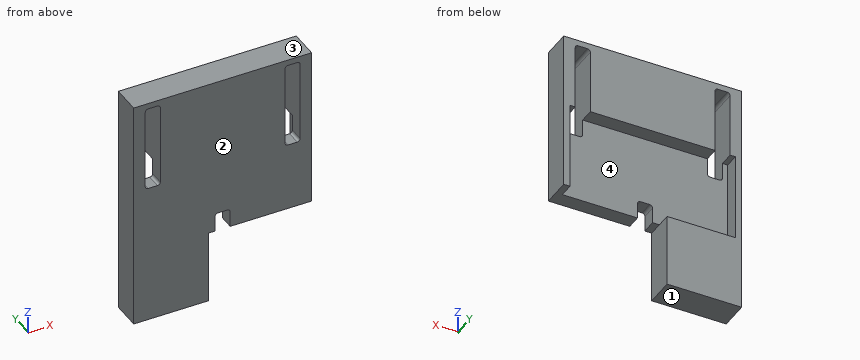
```python
from build123d import *

# Parameters (mm, degrees)
BOSS_EXTRUDE5_DEPTH = 10
CUT_EXTRUDE6_DEPTH  = 5
FILLET4_R           = 1
MIRROR25_DEPTH      = 10
MIRROR25_2_DEPTH    = 5
SKETCH20_W          = 35.925
SKETCH20_H          = 25.502594227
CUT_EXTRUDE7_DEPTH  = 10


# Read off the part's stored shape, not the designer's step: Mirror25
with BuildPart() as part:
    # Sketch15 → Boss-Extrude5 (new body)
    with BuildSketch(Plane(origin=(0, 0, 0), x_dir=(1, 0, 0), z_dir=(0, 1, 0))):
        Polygon((24.3, 76.900659127), (-6.625, 76.900659127), (-6.625, -4.5), (24.3, -4.5), (24.3, 44.900659127), (21.675, 44.900659127), (21.675, 47.400659127), (21.675, 72.400659127), (21.675, 74.900659127), (24.3, 74.900659127), align=None)
        Polygon((-2.625, 25), (-2.625, 0), (-2.625, -2.5), (0, -2.5), (2.625, -2.5), (2.625, 0), (2.625, 25), (2.625, 27.5), (0, 27.5), (-2.625, 27.5), align=None, mode=Mode.SUBTRACT)
    extrude(amount=BOSS_EXTRUDE5_DEPTH)

    # Sketch18 → Cut-Extrude6 (cut)
    with BuildSketch(Plane(origin=(0, 10, 0), x_dir=(1, 0, 0), z_dir=(0, 1, 0))):
        Polygon((21.675, 51.3980649), (-4.44053483, 51.3980649), (-4.44053483, 20.8980649), (24.3, 20.8980649), (24.3, 51.3980649), align=None)
    extrude(amount=-CUT_EXTRUDE6_DEPTH, mode=Mode.SUBTRACT)

    # Fillet4
    fillet4_edges = [part.edges().sort_by_distance(p)[0] for p in [
        (21.675, 5, -74.900659127),
        (-2.625, 5, 2.5),
        (2.625, 5, 2.5),
        (2.625, 2.5, -27.5),
        (-2.625, 2.5, -27.5),
        (21.675, 2.5, -44.900659127),
    ]]
    fillet(fillet4_edges, radius=FILLET4_R)

    # Mirror25 outline → Mirror25 (add)
    with BuildSketch(Plane(origin=(0, 0, 0), x_dir=(1, 0, 0), z_dir=(0, 1, 0))):
        with BuildLine():
            Line((45.975, 20.8980649), (24.3, 20.8980649))
            Line((24.3, 20.8980649), (24.3, -4.5))
            Line((24.3, -4.5), (55.225, -4.5))
            Line((55.225, -4.5), (55.225, 76.900659127))
            Line((55.225, 76.900659127), (24.3, 76.900659127))
            Line((24.3, 76.900659127), (24.3, 74.900659127))
            Line((24.3, 74.900659127), (25.925, 74.900659127))
            ThreePointArc((25.925, 74.900659127), (26.632106781, 74.607765908), (26.925, 73.900659127))
            Line((26.925, 73.900659127), (26.925, 51.3980649))
            Line((26.925, 51.3980649), (53.04053483, 51.3980649))
            Line((53.04053483, 51.3980649), (53.04053483, 20.8980649))
            Line((53.04053483, 20.8980649), (51.225, 20.8980649))
            Line((51.225, 20.8980649), (51.225, -1.5))
            ThreePointArc((51.225, -1.5), (50.932106781, -2.207106781), (50.225, -2.5))
            Line((50.225, -2.5), (46.975, -2.5))
            ThreePointArc((46.975, -2.5), (46.267893219, -2.207106781), (45.975, -1.5))
            Line((45.975, -1.5), (45.975, 20.8980649))
        make_face()
    extrude(amount=MIRROR25_DEPTH)

    # Mirror25 2 outline → Mirror25 2 (add)
    with BuildSketch(Plane(origin=(0, 0, 0), x_dir=(1, 0, 0), z_dir=(0, 1, 0))):
        with BuildLine():
            Line((25.925, 44.900659127), (24.3, 44.900659127))
            Line((24.3, 44.900659127), (24.3, 20.8980649))
            Line((24.3, 20.8980649), (45.975, 20.8980649))
            Line((45.975, 20.8980649), (45.975, 26.5))
            ThreePointArc((45.975, 26.5), (46.267893219, 27.207106781), (46.975, 27.5))
            Line((46.975, 27.5), (50.225, 27.5))
            ThreePointArc((50.225, 27.5), (50.932106781, 27.207106781), (51.225, 26.5))
            Line((51.225, 26.5), (51.225, 20.8980649))
            Line((51.225, 20.8980649), (53.04053483, 20.8980649))
            Line((53.04053483, 20.8980649), (53.04053483, 51.3980649))
            Line((53.04053483, 51.3980649), (26.925, 51.3980649))
            Line((26.925, 51.3980649), (26.925, 45.900659127))
            ThreePointArc((26.925, 45.900659127), (26.632106781, 45.193552346), (25.925, 44.900659127))
        make_face()
    extrude(amount=MIRROR25_2_DEPTH)

    # Sketch20 → Cut-Extrude7 (cut)
    with BuildSketch(Plane(origin=(0, 10, 0), x_dir=(1, 0, 0), z_dir=(0, 1, 0))):
        with Locations((37.2625, 64.149362014)):
            Rectangle(SKETCH20_W, SKETCH20_H)
    extrude(amount=-CUT_EXTRUDE7_DEPTH, mode=Mode.SUBTRACT)


solid = part.part
```
Could you check a few things on this model? Use its own coordinates, in mm. Face numbers are marked on the shaded views. Coordinates: 2 decimals unless noted, no trailing zeros. Write each loop counter-clockwise with the first axis right and the second up, starting at its lowest first coordinate (ties: lowest second). Pieces come first, ordered by that corner, then holes. Notation, with made-up numbers: (12, 15) - (20, 15) arc R21 ccw to (20, 33) - close; hole circle Ø9 at (-2, 5.5). An arc over 180 degrees is marked (long way). Use a Markdown table: item, result.
Q1. Thinking about a two-plate mould opening in Z: for the marked faces 1, 2, 3 and 4, which applies, +Z half, -Z half, draft (parallel to the pull), parting line (faces both ways), or undercut?
Geometry check:
| item | result |
|---|---|
| face 1 | -Z half |
| face 2 | draft |
| face 3 | +Z half |
| face 4 | undercut |
Q2. Please list where these lines run through material, in increasing order: L1, parallel to X at y = 1.5, z = -13 (3 decimals); L2, parallel to Z at x = 47, y = 1.25; L3, parallel to Z at x = 0, y = 1.75.
Geometry check:
| item | result |
|---|---|
| L1 | x = -6.625 to -2.625, 2.625 to 45.975, 51.225 to 55.225 |
| L2 | z = -51.4 to -27.5, 2.5 to 4.5 |
| L3 | z = -76.9 to -27.5, 2.5 to 4.5 |
Q3. Imagine slicing it at A-A (z = -23). List the corners of the cut face in (x, y) for me (3 decimals), and give its area (3 significant figures).
Geometry check:
| item | result |
|---|---|
| outline | (-6.625, 0) - (-2.625, 0) - (-2.625, 5) - (-4.441, 5) - (-4.441, 10) - (-6.625, 10) - close; (2.625, 0) - (45.975, 0) - (45.975, 5) - (2.625, 5) - close; (51.225, 0) - (55.225, 0) - (55.225, 10) - (53.041, 10) - (53.041, 5) - (51.225, 5) - close |
| area | 279 mm2 |
Q4. Imagine slicing it at D-D (z = -44). List the corners of the cut face in (x, y) for me (3 decimals).
Geometry check:
| item | result |
|---|---|
| outline | (-6.625, 0) - (55.225, 0) - (55.225, 10) - (53.041, 10) - (53.041, 5) - (-4.441, 5) - (-4.441, 10) - (-6.625, 10) - close |
Q5. Imagine slicing it at B-B (y = 1.25). List the corners of the cut face in (x, z) for me (3 decimals), and give its area (3 significant figures).
Geometry check:
| item | result |
|---|---|
| outline | (-6.625, -76.901) - (19.3, -76.901) - (19.3, -51.398) - (21.675, -51.398) - (21.675, -45.901) arc R1 cw to (22.675, -44.901) - (25.925, -44.901) arc R1 cw to (26.925, -45.901) - (26.925, -51.398) - (55.225, -51.398) - (55.225, 4.5) - (-6.625, 4.5) - close; hole (-2.625, -26.5) arc R1 ccw to (-1.625, -27.5) - (1.625, -27.5) arc R1 ccw to (2.625, -26.5) - (2.625, 1.5) arc R1 ccw to (1.625, 2.5) - (-1.625, 2.5) arc R1 ccw to (-2.625, 1.5) - close; hole (45.975, -26.5) arc R1 ccw to (46.975, -27.5) - (50.225, -27.5) arc R1 ccw to (51.225, -26.5) - (51.225, 1.5) arc R1 ccw to (50.225, 2.5) - (46.975, 2.5) arc R1 ccw to (45.975, 1.5) - close |
| area | 3,770 mm2 |
Q6. Imagine slicing it at C-C (x = 16.5). List the corners of the cut face in (y, z) for me.
Geometry check:
| item | result |
|---|---|
| outline | (0, -76.9) - (10, -76.9) - (10, -51.4) - (5, -51.4) - (5, -20.9) - (10, -20.9) - (10, 4.5) - (0, 4.5) - close |
Q7. I'm going to push flat-ended pins straight in: pin 1 Ø3 at (y, z) = (6.5, -64.5) entering from +X; pin 2 Ø3 at (x, y) = (35, 4.5) entering from -Z; pin 3 Ø1.5 at (x, y) = (52, 8) entering from -Z. Where does each tip first touch, or does it pass through?
Geometry check:
| item | result |
|---|---|
| pin 1 | stops at x = 19.3 |
| pin 2 | stops at z = -51.4 |
| pin 3 | stops at z = -20.9 |
